Work out the finished part from the listing and answer in its coordinate system (mm). A direction names the side the tool comes from. Coordinates: 2 decimals unless noted, no trailing zeros. Order: outer loops, then holes, each group sorted by start corner. A loop starts at its lowest first (then second) coordinate and runs counter-clockwise, first axis right, second up. Notation, with made-up numbers: M 88.25,-24.5 L 110.25,-24.5 A4 cw 110.25,-17.5 Z; hole C 7.25,10.25 d4. An arc over 180 degrees is marked long. Use a Markdown table: item, result. Add a question column.
from build123d import *

# Parameters (mm, degrees)
SKETCH_1_R             = 60
EXTRUDE_1_DEPTH        = 100
HOLE_WIZARD_M8_1_D     = 6.8
HOLE_WIZARD_M8_1_DEPTH = 22.25
HOLE_WIZARD_M8_1_TIP   = 2.042926105


with BuildPart() as part:
    # 草圖1 → 填料-伸長1 (new body)
    with BuildSketch(Plane(origin=(0, 0, 0), x_dir=(1, 0, 0), z_dir=(0, 1, 0))):
        Circle(SKETCH_1_R)
    extrude(amount=EXTRUDE_1_DEPTH)

    # M8 螺紋孔1
    with Locations(Plane(origin=(0, 100, -40), x_dir=(0, 0, 1), z_dir=(0, 1, 0))):
        with Locations((0, 0), (15.060407926, 31.273259299), (48.900837358, 38.997116487), (76.038754716, 17.355349565), (76.038754716, -17.355349565), (48.900837358, -38.997116487), (15.060407926, -31.273259299)):
            Hole(HOLE_WIZARD_M8_1_D / 2, depth=HOLE_WIZARD_M8_1_DEPTH)
            with Locations((0, 0, -(HOLE_WIZARD_M8_1_DEPTH + HOLE_WIZARD_M8_1_TIP / 2))):  # 118° drill point
                Cone(0, HOLE_WIZARD_M8_1_D / 2, HOLE_WIZARD_M8_1_TIP, mode=Mode.SUBTRACT)


solid = part.part
(1) A cutting plane is placed at B-B on x = -24.5. Write down the section's boundary in (y, z), plus the area to 3 significant figures.
(2) Given P1, Ø5, axis at x = 33.5, y = 47, coming from the +Z side; P2, Ø4, axis at x = -39, z = 8.9, coming from the +Y side; P3, Ø1, axis at y = 44, z = 31, coming from the -X side, each flat-ended and moving along its own axis, determine where each tip first touches the part or whether it passes through.
(3) Which of the six approach directions +Z, -Z, +X, -X, +Y, -Y give full straight-line access (tool end or side, diameter ignored) to faces 4 (the flat face through (-1, 100, -1)), 5 (the cylindrical face through (35.68, 88.72, 9.64))?
(4) Straight lines are drawn through the part: line 1 (X direction, y = 95.25, z = -40); line 2 (Z direction, x = 42, y = 86); line 3 (Z direction, x = -11.5, y = 32.5). For each, find the intervals that lie inside material, in ascending order.
(5) The mould has two halves that part along Z. Classify faces 1 (the cylindrical face through (-59.94, 49.3, -2.64)), 2 (the cylindrical face through (16.05, 88.72, 32.9)), 3 (the flat face through (-1, 0, -1)): pulls with the +Z half, pulls with the -Z half, needs draft (parallel to the pull), parting line crosses it, or undercut.
(6) A cutting plane is placed at C-C on z = -49. Write down the section's boundary in (x, y), plus the area to 3 significant figures.
(7) A cutting plane is placed at A-A on y = 12.5. Write down the section's boundary in (x, z), plus the area to 3 significant figures.
From the geometry:
| question | item | result |
|---|---|---|
| 1 | outline | M 0,-54.77 L 100,-54.77 L 100,54.77 L 0,54.77 Z |
| 1 | area | 11,000 mm2 |
| 2 | P1 | stops at z = 51.37 |
| 2 | P2 | stops at y = 76.91 |
| 2 | P3 | stops at x = -51.67 |
| 3 | face 4 | +Z, -Z, +X, -X, +Y |
| 3 | face 5 | +Y |
| 4 | line 1 | x = -44.72 to -3.4, 3.4 to 44.72 |
| 4 | line 2 | z = -42.85 to 7.31, 10.5 to 42.85 |
| 4 | line 3 | z = -58.89 to 58.89 |
| 5 | face 1 | parting line crosses it |
| 5 | face 2 | undercut |
| 5 | face 3 | needs draft |
| 6 | outline | M -34.63,0 L 34.63,0 L 34.63,100 L -34.63,100 Z |
| 6 | area | 6,930 mm2 |
| 7 | outline | C 0,0 d120 |
| 7 | area | 11,300 mm2 |
